For this review, take the finished solid that the model builds, in its own axes (mm). Coordinates: 2 decimals unless noted, no trailing zeros. Loops run counter-clockwise (first coordinate to the right, second up) from the corner with the lowest first, then second, coordinate; pieces in that order, holes last. Notation, with made-up numbers: (20, 18.5) - (49, 18.5) arc R25 cw to (49, 57.5) - close; hole circle Ø9 at (30.5, 87.5). An arc over 180 degrees is marked (long way). One line per item, written item: value. Start each with the question number.
1. Take a section at D-D, the plane x = 49. State the section outline as (y, z) points.
2. To check wall thickness, follow line 1 (X direction, y = 0.1, z = 0); line 2 (X direction, y = -0.9, z = 22.15); line 3 (Z direction, x = -30.5, y = 0.2). State the ranges of each line that lie inside material, in increasing order. Write a range as from..to.
3. Take a section at C-C, the plane y = 0.5. Count the separate pieces of the cut face and the enclosed holes in it, and give its area (3 significant figures).
4. Insertion check: pin 1 (1 mm diameter, centred on x = 18, y = 0.5, fed in from +Z); pin 2 (1.5 mm diameter, centred on y = 0.5, z = -52, fed in from +X); pin 3 (0.9 mm diameter, centred on x = 51.5, y = -0.5, fed in from +Z). Each pin has a flat end and moves straight along its axis. Give the tip position at first contact, or say it passes through.
5. Take a section at B-B, the plane z = -22.15. State the section outline as (x, y) points.
6. Take a section at A-A, the plane x = 30.5. State the section outline as (y, z) points, and give its area (3 significant figures).
```python
from build123d import *

# Parameters (mm, degrees)
ESBO_O1_W                = 140
ESBO_O1_H                = 100
RESSALTO_EXTRUS_O1_DEPTH = 1.5
RESSALTO_EXTRUS_O2_DEPTH = 3
ESBO_O2_R                = 1.5
CORTE_EXTRUS_O1_DEPTH    = 4
SKETCH1_R                = 1.7
CUT_EXTRUDE1_DEPTH       = 1
CUT_EXTRUDE1_DEPTH_BACK  = 4
SKETCH2_W                = 3.2
SKETCH2_H                = 15.2
CUT_EXTRUDE3_DEPTH       = 2.5
CUT_EXTRUDE3_DEPTH_BACK  = 2.5


with BuildPart() as part:
    # Esboço1 → Ressalto-extrusão1 (new body, symmetric)
    with BuildSketch(Plane(origin=(0, 0, 0), x_dir=(1, 0, 0), z_dir=(0, 1, 0))):
        Rectangle(ESBO_O1_W, ESBO_O1_H)
    extrude(amount=RESSALTO_EXTRUS_O1_DEPTH, both=True)

    # Esboço4 → Ressalto-extrusão2 (add, through all)
    with BuildSketch(Plane(origin=(0, 1.5, 0), x_dir=(1, 0, 0), z_dir=(0, 1, 0))):
        with BuildLine():
            Line((6.5, 53), (20, 53))
            Line((20, 53), (20, 50))
            Line((20, 50), (-20, 50))
            Line((-20, 50), (-20, 53))
            Line((-20, 53), (-6.5, 53))
            ThreePointArc((-6.5, 53), (-5.085786438, 53.585786438), (-4.5, 55))
            Line((-4.5, 55), (-4.5, 56))
            Line((-4.5, 56), (4.5, 56))
            Line((4.5, 56), (4.5, 55))
            ThreePointArc((4.5, 55), (5.085786438, 53.585786438), (6.5, 53))
        make_face()
        with BuildLine():
            Line((-76, 4.5), (-76, -4.5))
            Line((-76, -4.5), (-75, -4.5))
            ThreePointArc((-75, -4.5), (-73.585786438, -5.085786438), (-73, -6.5))
            Line((-73, -6.5), (-73, -20))
            Line((-73, -20), (-70, -20))
            Line((-70, -20), (-70, 20))
            Line((-70, 20), (-73, 20))
            Line((-73, 20), (-73, 6.5))
            ThreePointArc((-73, 6.5), (-73.585786438, 5.085786438), (-75, 4.5))
            Line((-75, 4.5), (-76, 4.5))
        make_face()
        with BuildLine():
            Line((4.5, -56), (4.5, -55))
            ThreePointArc((4.5, -55), (5.085786438, -53.585786438), (6.5, -53))
            Line((6.5, -53), (20, -53))
            Line((20, -53), (20, -50))
            Line((20, -50), (-20, -50))
            Line((-20, -50), (-20, -53))
            Line((-20, -53), (-6.5, -53))
            ThreePointArc((-6.5, -53), (-5.085786438, -53.585786438), (-4.5, -55))
            Line((-4.5, -55), (-4.5, -56))
            Line((-4.5, -56), (4.5, -56))
        make_face()
        with BuildLine():
            Line((70, 20), (73, 20))
            Line((73, 20), (73, 6.5))
            ThreePointArc((73, 6.5), (73.585786438, 5.085786438), (75, 4.5))
            Line((75, 4.5), (76, 4.5))
            Line((76, 4.5), (76, -4.5))
            Line((76, -4.5), (75, -4.5))
            ThreePointArc((75, -4.5), (73.585786438, -5.085786438), (73, -6.5))
            Line((73, -6.5), (73, -20))
            Line((73, -20), (70, -20))
            Line((70, -20), (70, 20))
        make_face()
    extrude(amount=-RESSALTO_EXTRUS_O2_DEPTH)

    # Esboço2 → Corte-extrusão1 (cut, through all)
    with BuildSketch(Plane(origin=(0, 1.5, 0), x_dir=(1, 0, 0), z_dir=(0, 1, 0))):
        with Locations((0, -51.5)):
            Circle(ESBO_O2_R)
        with Locations((0, 51.5)):
            Circle(ESBO_O2_R)
        with Locations((71.5, 0)):
            Circle(ESBO_O2_R)
        with Locations((-71.5, 0)):
            Circle(ESBO_O2_R)
    extrude(amount=-CORTE_EXTRUS_O1_DEPTH, mode=Mode.SUBTRACT)

    # Sketch1 → Cut-Extrude1 (cut, two sides)
    with BuildSketch(Plane(origin=(0, 1.5, 0), x_dir=(1, 0, 0), z_dir=(0, 1, 0))) as cut_extrude1_sk:
        with Locations((30.5, -22.15)):
            Circle(SKETCH1_R)
        with Locations((37.9, -22.15)):
            Circle(SKETCH1_R)
        with Locations((37.9, 22.15)):
            Circle(SKETCH1_R)
        with Locations((30.5, 22.15)):
            Circle(SKETCH1_R)
        with Locations((-30.5, 22.15)):
            Circle(SKETCH1_R)
        with Locations((-37.9, 22.15)):
            Circle(SKETCH1_R)
        with Locations((-37.9, -22.15)):
            Circle(SKETCH1_R)
        with Locations((-30.5, -22.15)):
            Circle(SKETCH1_R)
    extrude(amount=CUT_EXTRUDE1_DEPTH, mode=Mode.SUBTRACT)
    extrude(cut_extrude1_sk.sketch, amount=-CUT_EXTRUDE1_DEPTH_BACK, mode=Mode.SUBTRACT)

    # Sketch2 → Cut-Extrude3 (cut, two sides)
    with BuildSketch(Plane(origin=(0, 0, 0), x_dir=(1, 0, 0), z_dir=(0, 1, 0))) as cut_extrude3_sk:
        with Locations((61.4, 0)):
            Rectangle(SKETCH2_W, SKETCH2_H)
    extrude(amount=CUT_EXTRUDE3_DEPTH, mode=Mode.SUBTRACT)
    extrude(cut_extrude3_sk.sketch, amount=-CUT_EXTRUDE3_DEPTH_BACK, mode=Mode.SUBTRACT)


solid = part.part
```
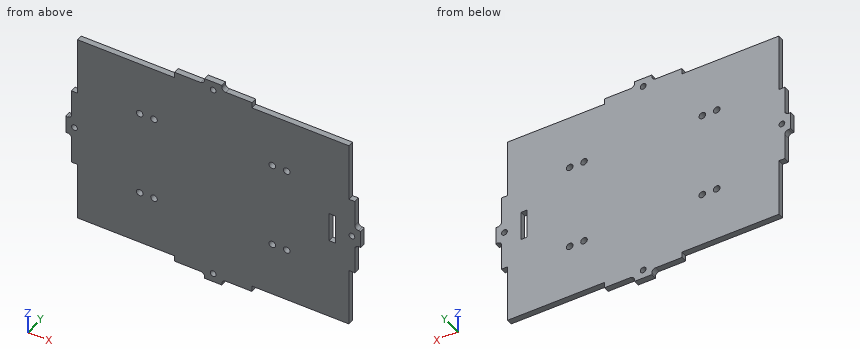
Solutions:
1. outline: (-1.5, -50) - (1.5, -50) - (1.5, 50) - (-1.5, 50) - close
2. line 1: -76..-73, -70..59.8, 63..70, 73..76
2. line 2: -70..-39.6, -36.2..-32.2, -28.8..28.8, 32.2..36.2, 39.6..70
2. line 3: -50..-23.85, -20.45..20.45, 23.85..50
3. separate pieces: 1
3. enclosed holes: 13
3. area: 14,400 mm2
4. pin 1: z = 53
4. pin 2: x = 20
4. pin 3: z = 50
5. outline: (-70, -1.5) - (-39.6, -1.5) - (-39.6, 1.5) - (-70, 1.5) - close; (-36.2, -1.5) - (-32.2, -1.5) - (-32.2, 1.5) - (-36.2, 1.5) - close; (-28.8, -1.5) - (28.8, -1.5) - (28.8, 1.5) - (-28.8, 1.5) - close; (32.2, -1.5) - (36.2, -1.5) - (36.2, 1.5) - (32.2, 1.5) - close; (39.6, -1.5) - (70, -1.5) - (70, 1.5) - (39.6, 1.5) - close
6. outline: (-1.5, -50) - (1.5, -50) - (1.5, -23.85) - (-1.5, -23.85) - close; (-1.5, -20.45) - (1.5, -20.45) - (1.5, 20.45) - (-1.5, 20.45) - close; (-1.5, 23.85) - (1.5, 23.85) - (1.5, 50) - (-1.5, 50) - close
6. area: 280 mm2
